Autodesk Inventor part; units mm, degrees
ref_plane "工作平面1" through (0, 0, 0) normal (0, 0, 1) x (1, 0, 0)
ref_plane "工作平面3" through (-5.8702, 48.2125, -2.9174) normal (-0.9999955, 0, 0.0030077) x (0.0030077, 0, 0.9999955)
ref_plane "工作平面4" through (0.1, 52.2125, 8.4448) normal (1, 0, 0) x (0, 1, 0)
ref_plane "工作平面1" through (0, 0, 0) normal (0, 0, 1) x (1, 0, 0)
sketch "草圖1" plane through (0, 0, 0) normal (0, 0, 1) x (1, 0, 0)
  circle A0 centre (-7.075, 38.25) radius 2.165
  circle A1 centre (7.075, 38.25) radius 2.165
  arc A2 (-15.075, -26.25) -> (-13.075, -28.25) centre (-13.075, -26.25) ccw
  line L0 (-13.075, -28.25) -> (13.075, -28.25)
  arc A3 (13.075, -28.25) -> (15.075, -26.25) centre (13.075, -26.25) ccw
  line L1 (15.075, -26.25) -> (15.075, 43.25) construction
  line L2 (-15.075, 43.25) -> (15.075, 43.25) construction
  line L3 (-15.075, 43.25) -> (-15.075, -26.25) construction
  line L4 (-10.075, 23.25) -> (10.075, 23.25)
  line L5 (10.075, 23.25) -> (10.075, 3.1)
  line L6 (10.075, 3.1) -> (-10.075, 3.1)
  line L7 (-10.075, 3.1) -> (-10.075, 23.25)
  line L8 (-10.075, -3.1) -> (10.075, -3.1)
  line L9 (10.075, -3.1) -> (10.075, -23.25)
  line L10 (10.075, -23.25) -> (-10.075, -23.25)
  line L11 (-10.075, -23.25) -> (-10.075, -3.1)
  arc A4 (7.075, 33.585) -> (7.075, 42.915) centre (7.075, 38.25) ccw
  arc A5 (-7.075, 42.915) -> (-7.075, 33.585) centre (-7.075, 38.25) ccw
  line L12 (7.075, 33.585) -> (-7.075, 33.585)
  line L13 (7.075, 42.915) -> (-7.075, 42.915)
  circle A6 centre (7.075, 38.25) radius 1.6
  circle A7 centre (-7.075, 38.25) radius 1.6
  point P0 (0, 0)
  dimension "d0" = 2.5
  dimension "d1" = 2.5
  dimension "d20" = 3.2
  dimension "d21" = 3.2
extrude "擠出1" add sketch "草圖1" along normal blind 2 contours A0 | A1 | L12 A5 L13 A4
ref_plane "工作平面3" through (-5.8702, 48.2125, -2.9174) normal (-0.9999955, 0, 0.0030077) x (0.0030077, 0, 0.9999955)
ref_plane "工作平面4" through (0.1, 52.2125, 8.4448) normal (1, 0, 0) x (0, 1, 0)
sketch "草圖3" plane through (0.1, 52.2125, 8.4448) normal (1, 0, 0) x (0, 1, 0)
  line L0 (-18.6275, -8.4448) -> (-9.2975, -8.4448)
  line L1 (-9.2975, -8.4448) -> (-9.2975, -6.4448)
  line L2 (-18.6275, -6.4448) -> (-9.2975, -6.4448)
  line L3 (-18.6275, -8.4448) -> (-18.6275, -6.4448)
  line L4 (4, -7.96) -> (4, 0)
  line L5 (4, 0) -> (0, 0)
  line L6 (0, 0) -> (0, -9.8)
  line L7 (12.94, -9.8) -> (0, -9.8)
  line L8 (12.94, -9.8) -> (12.94, 0)
  line L9 (12.94, 0) -> (8.94, 0)
  line L10 (8.94, 0) -> (8.94, -7.96)
  line L11 (8.94, -7.96) -> (4, -7.96)
  line L12 (-9.2975, -6.4448) -> (-9.2975, 1.5)
  line L13 (-9.2975, 1.5) -> (5.4231, 1.5)
  line L14 (5.4231, 1.5) -> (5.4231, -6)
  line L15 (5.4231, -6) -> (7.4231, -6)
  line L16 (7.4231, -6) -> (7.4231, 3.5)
  line L17 (7.4231, 3.5) -> (-11.2975, 3.5)
  line L18 (-11.2975, 3.5) -> (-11.2975, -6.4448)
  point P0 (-52.2125, -8.4448)
  point P1 (-9.2975, 3.5)
  dimension "d12" = 2
  dimension "d13" = 2
  dimension "d14" = 2
  dimension "d15" = 1.5
  dimension "d16" = 7.5
extrude "擠出3" add sketch "草圖3" against normal blind 6.1 contours L2 L18 L17 L16 L15 L14 L13 L12
fillet "圓角1" radius 2 3 edges at (0.1, 41.915, 2) (-2.95, 40.915, 2) (-6, 41.915, 2)
properties part number "j3 endstop blocker_3D 列印"
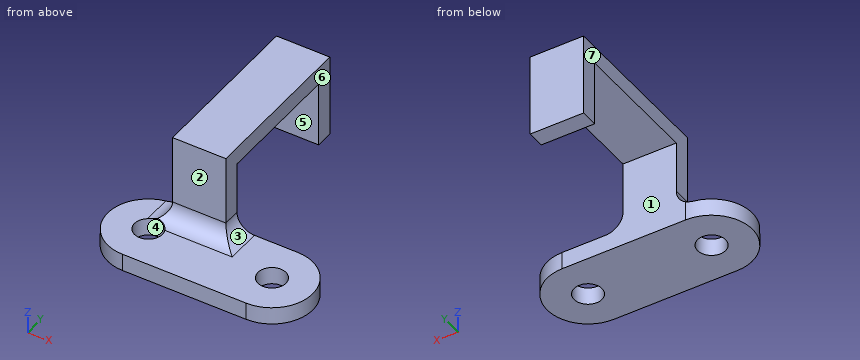
Build history of the part. All positions in model axes, mm. Face numbers are marked on the shaded views. A direction names the side the tool comes from. Round coordinates to 2 decimals unless told otherwise and drop trailing zeros. Loops run counter-clockwise (first coordinate to the right, second up) from the corner with the lowest first, then second, coordinate; pieces in that order, holes last. Notation, with made-up numbers: (-12, 80.25) -> (40, 80.25) arc R18 ccw to (40, 95.25) -> close; hole circle Ø6 at (-4.75, -18.75). An arc over 180 degrees is marked (long way). Use CSV: the item, a comma, the result in double quotes. Start each with the question number.
Q1. Saw through at A-A on z = 9.25. Give the cut face in (x, y) (3 decimals), and give its area (3 significant figures).
Q2. Saw through at C-C on x = 2.5. Give the cut face in (y, z) (3 decimals).
Q3. Mould opens along X. For the marked faces 4, 5, 6 and 7 say: +X half, -X half, draft (parallel to the pull), parting line (faces both ways), or undercut.
Q4. Which spindle directions (+Z, -Z, +X, -X, +Y, -Y) get a long thin tool onto all of the face, cutting with end or side? Do the marked faces 1, 2 and 3. Say none if no direction does.
Q5. Flat gauge pins, fed straight in: pin 1 Ø6 at (x, z) = (8, 2) entering from +Y (3 decimals); pin 2 Ø1.5 at (x, z) = (-1, 4.5) entering from -Y; pin 3 Ø1 at (x, y) = (-4, 59) entering from -Z. Where does each tip first touch, or does it go through?
Q6. Drill centre lines: L1, parallel to Y at x = -1.5, z = 5 (3 decimals); L2, parallel to Z at x = 1, y = 38; L3, parallel to Z at x = -1, y = 49. Where is each one in solid material? Low to high.
Q7. Saw through at D-D on y = 50.75. Give the cut face in (x, z), and give its area (3 significant figures).
Q8. Saw through at B-B on y = 38.25. Give the cut face in (x, z) (3 decimals).
Solutions:
1,outline,"(-6, 40.915) -> (0.1, 40.915) -> (0.1, 42.915) -> (-6, 42.915) -> close; (-6, 57.636) -> (0.1, 57.636) -> (0.1, 59.636) -> (-6, 59.636) -> close"
1,area,"24.4 mm^2"
2,outline,"(33.585, 0) -> (42.915, 0) -> (42.915, 2) -> (33.585, 2) -> close"
3,face 4,"undercut"
3,face 5,"draft"
3,face 6,"+X half"
3,face 7,"-X half"
4,face 1,"-Z, +X, -X"
4,face 2,"+Z, +X, -X, -Y"
4,face 3,"+Z, +X, +Y, -Y"
5,pin 1,"stops at y = 42.915"
5,pin 2,"stops at y = 40.9"
5,pin 3,"stops at z = 2.44"
6,L1,"y = 40.915 to 42.915, 57.636 to 59.636"
6,L2,"z = 0 to 2"
6,L3,"z = 9.94 to 11.94"
7,outline,"(-6, 9.94) -> (0.1, 9.94) -> (0.1, 11.94) -> (-6, 11.94) -> close"
7,area,"12.2 mm^2"
8,outline,"(-11.74, 0) -> (-8.675, 0) -> (-8.675, 2) -> (-11.74, 2) -> close; (-5.475, 0) -> (5.475, 0) -> (5.475, 2) -> (-5.475, 2) -> close; (8.675, 0) -> (11.74, 0) -> (11.74, 2) -> (8.675, 2) -> close"
